```python
from build123d import *

# Parameters (mm, degrees)
F0_W     = 3.1506001928
F0_H     = 3.9233311644
F0_W_2   = 15.8593781031
F0_W_3   = 15.828302058
F2_DEPTH = 25
F1_R     = 1.5
F3_DEPTH = 6
F4_DEPTH = 6


with BuildPart() as f2:
    # F0 (on Front) → F2 (new body)
    with BuildSketch(Plane.XZ):
        with BuildLine():
            ThreePointArc((5, 8.5672423611), (-2.9194014288, 12.6264412103), (-1.5908381189, 3.827069993))
            Line((-1.5908381189, 3.827069993), (-1.5908381189, 8.5672423611))
            Line((-1.5908381189, 8.5672423611), (1.5597620739, 8.5672423611))
            Line((1.5597620739, 8.5672423611), (1.5597620739, 3.8167537259))
            ThreePointArc((1.5597620739, 3.8167537259), (4.049617906, 5.6345652879), (5, 8.5672423611))
        make_face()
        with BuildLine():
            Line((-1.5908381189, 8.5672423611), (-1.5908381189, 3.827069993))
            ThreePointArc((-1.5908381189, 3.827069993), (-0.0163718198, 3.5672691648), (1.5597620739, 3.8167537259))
            Line((1.5597620739, 3.8167537259), (1.5597620739, 8.5672423611))
            Line((1.5597620739, 8.5672423611), (-1.5908381189, 8.5672423611))
        make_face()
        with Locations((-0.0155380225, 0)):
            Rectangle(F0_W, F0_H)
        with BuildLine():
            Line((-1.5908381189, 3.827069993), (-1.5908381189, 1.9616655822))
            Line((-1.5908381189, 1.9616655822), (1.5597620739, 1.9616655822))
            Line((1.5597620739, 1.9616655822), (1.5597620739, 3.8167537259))
            ThreePointArc((1.5597620739, 3.8167537259), (-0.0163718198, 3.5672691648), (-1.5908381189, 3.827069993))
        make_face()
        with Locations((9.4894511254, 0)):
            Rectangle(F0_W_2, F0_H)
        with Locations((-9.5049891479, 0)):
            Rectangle(F0_W_3, F0_H)
    extrude(amount=-F2_DEPTH)

    # F1 (on Top) → F3 (cut, symmetric)
    with BuildSketch(Plane.XY):
        with Locations((14.419140177, 6.4654615708)):
            Circle(F1_R)
    extrude(amount=F3_DEPTH, both=True, mode=Mode.SUBTRACT)

    # F1 (on Top) → F4 (cut, symmetric)
    with BuildSketch(Plane.XY):
        with Locations((-14.419140177, 6.4020673744)):
            Circle(F1_R)
    extrude(amount=F4_DEPTH, both=True, mode=Mode.SUBTRACT)


solid = f2.part
```
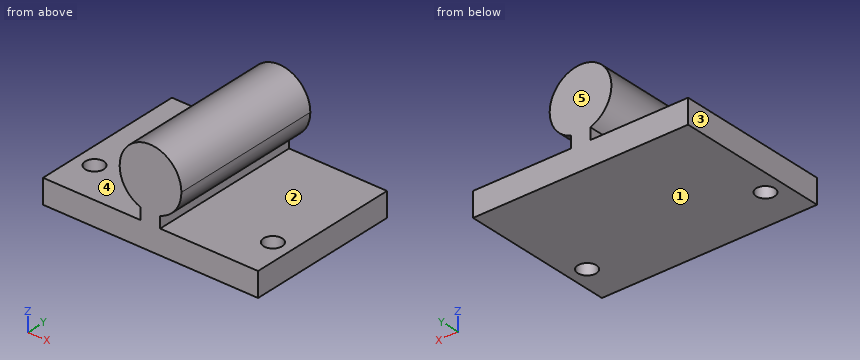
Can you work these out from the model? Positions are in its coordinate system, mm. Face numbers are marked on the shaded views. A direction names the side the tool comes from. Give positions to 0.01 mm unless a question says otherwise; leave off trailing zeros. Order: outer loops, then holes, each group sorted by start corner. A loop starts at its lowest first (then second) coordinate and runs counter-clockwise, first axis right, second up. Notation, with made-up numbers: (-34.5, 28.25) - (-3.5, 28.25) arc R14 cw to (-3.5, 47.25) - close; hole circle Ø1 at (6.25, 73). An arc over 180 degrees is marked (long way). Use a Markdown table: item, result. Add a question column.
Q1. On a 3-axis mill with a long thin cutter (end or side, diameter ignored), from which of +Z, -Z, +X, -X, +Y, -Y can I reach the whole of each face in a straight line? I mean the marked faces 4 and 5. Say none if no direction works.
Q2. If we section it at D-D on z = 1.5: Write out the boundary of the cut face in (x, y), plus the area to 3 significant figures.
Q3. If we section it at A-A on x = -3.5: Write out the boundary of the cut face in (y, z), plus the area to 3 significant figures.
Q4. If we mould it in two halves opening along Z, with no side actions, what happens to the marked faces 1, 2 and 3? For each: released by +Z, released by -Z, zero draft, split by the parting line, or undercut.
Q5. I'm going to push flat-ended pins straight in: pin 1 (0.6 mm diameter, centred on y = 10.5, z = 3, fed in from +X); pin 2 (2 mm diameter, centred on y = 14.5, z = 3, fed in from -X); pin 3 (5 mm diameter, centred on x = -14.42, y = 6.4, fed in from +Z). Where does each tip first touch, or does it pass through?
Q6. If we section it at C-C on y = 5.5: Write out the boundary of the cut face in (x, z), plus the area to 3 significant figures.
Q7. Please list where these lines run through material, in increasing order: line 1 along Z through (x, y) = (11, 8); line 2 along Z through (x, y) = (-2, 11.25); line 3 along X through (y, z) = (8.5, 3.25).
Q8. If we section it at B-B on y = 2.75: Write out the boundary of the cut face in (x, z).
Answers follow:
| question | item | result |
|---|---|---|
| 1 | face 4 | -X, +Y, -Y |
| 1 | face 5 | +Z, -Z, +X, -X, +Y |
| 2 | outline | (-17.42, 0) - (17.42, 0) - (17.42, 25) - (-17.42, 25) - close; hole circle Ø3 at (-14.42, 6.4); hole circle Ø3 at (14.42, 6.47) |
| 2 | area | 857 mm^2 |
| 3 | outline | (0, -1.96) - (25, -1.96) - (25, 1.96) - (0, 1.96) - close; (0, 5) - (25, 5) - (25, 12.14) - (0, 12.14) - close |
| 3 | area | 277 mm^2 |
| 4 | face 1 | released by -Z |
| 4 | face 2 | undercut |
| 4 | face 3 | zero draft |
| 5 | pin 1 | stops at x = 1.56 |
| 5 | pin 2 | stops at x = -2.03 |
| 5 | pin 3 | stops at z = 1.96 |
| 6 | outline | (-17.42, -1.96) - (-15.62, -1.96) - (-15.62, 1.96) - (-17.42, 1.96) - close; (-13.22, -1.96) - (13.27, -1.96) - (13.27, 1.96) - (1.56, 1.96) - (1.56, 3.82) arc R5 ccw (long way) to (-1.59, 3.83) - (-1.59, 1.96) - (-13.22, 1.96) - close; (15.57, -1.96) - (17.42, -1.96) - (17.42, 1.96) - (15.57, 1.96) - close |
| 6 | area | 202 mm^2 |
| 7 | line 1 | z = -1.96 to 1.96 |
| 7 | line 2 | z = -1.96 to 1.96, 3.98 to 13.15 |
| 7 | line 3 | x = -1.59 to 1.56 |
| 8 | outline | (-17.42, -1.96) - (17.42, -1.96) - (17.42, 1.96) - (1.56, 1.96) - (1.56, 3.82) arc R5 ccw (long way) to (-1.59, 3.83) - (-1.59, 1.96) - (-17.42, 1.96) - close |
